from build123d import *

# Parameters (mm, degrees)
SKETCH_1_R          = 25
EXTRUDE_1_DEPTH     = 25
SKETCH_2_R          = 17.5
CUT_EXTRUDE_1_DEPTH = 10
SKETCH_3_R          = 2.5
CUT_EXTRUDE_2_DEPTH = 39.405728739


with BuildPart() as part:
    # 草图1 → 凸台-拉伸1 (new body)
    with BuildSketch(Plane(origin=(0, 0, 0), x_dir=(1, 0, 0), z_dir=(0, 1, 0))):
        with Locations(Location((0, 0, 0), (0, 0, 270))):
            Circle(SKETCH_1_R)
    extrude(amount=EXTRUDE_1_DEPTH)

    # 草图2 → 切除-拉伸1 (cut)
    with BuildSketch(Plane.XZ):
        with Locations(Location((0, 0, 0), (0, 0, 270))):
            Circle(SKETCH_2_R)
    cut_extrude_1 = extrude(amount=-CUT_EXTRUDE_1_DEPTH, mode=Mode.SUBTRACT)

    # 镜向1: 切除-拉伸1 across plane
    add(cut_extrude_1.mirror(Plane(origin=(0, 12.5, 0), x_dir=(0, 0, 1), z_dir=(0, -1, 0))), mode=Mode.SUBTRACT)

    # 草图3 → 切除-拉伸2 (cut, through all)
    with BuildSketch(Plane.XZ.offset(-10)):
        with Locations(Location((0, 0, 0), (0, 0, 270))):
            Circle(SKETCH_3_R)
    extrude(amount=-CUT_EXTRUDE_2_DEPTH, mode=Mode.SUBTRACT)


solid = part.part
Verification items for the finished model (mm, model axes). A direction names the side the tool comes from. Coordinates: 2 decimals unless noted, no trailing zeros. Write each loop counter-clockwise with the first axis right and the second up, starting at its lowest first coordinate (ties: lowest second). Pieces come first, ordered by that corner, then holes. Notation, with made-up numbers: (52.25, 54.25) - (98.25, 54.25) arc R26 cw to (98.25, 86.25) - close; hole circle Ø8 at (45.5, 48.25). An arc over 180 degrees is marked (long way). Answer as a JSON object with one key per item and string values.
(1) Cross-section at B-B on x = 0. Record the cut outline in (y, z).
Report:
{"outline": "(0, -25) - (25, -25) - (25, -17.5) - (15, -17.5) - (15, -2.5) - (10, -2.5) - (10, -17.5) - (0, -17.5) - close; (0, 17.5) - (10, 17.5) - (10, 2.5) - (15, 2.5) - (15, 17.5) - (25, 17.5) - (25, 25) - (0, 25) - close"}
(2) Cross-section at C-C on y = 12.5. Record the cut outline in (x, z).
Report:
{"outline": "circle Ø50 at (0, 0); hole circle Ø5 at (0, 0)"}
(3) Cross-section at A-A on z = 0. Record the cut outline in (x, y), plus the area to 3 significant figures.
Report:
{"outline": "(-25, 0) - (-17.5, 0) - (-17.5, 10) - (-2.5, 10) - (-2.5, 15) - (-17.5, 15) - (-17.5, 25) - (-25, 25) - close; (2.5, 10) - (17.5, 10) - (17.5, 0) - (25, 0) - (25, 25) - (17.5, 25) - (17.5, 15) - (2.5, 15) - close", "area": "525 mm^2"}
(4) Tool access check on faces 4 (the flat face through (-5, 25, -17)), 5 (the cylindrical face through (-10.648, 4.93, 13.887)), 6 (the cylindrical face through (-10.648, 20.07, 13.887)). Record the directions out of +Z, -Z, +X, -X, +Y, -Y that give a thin tool (end or side, any length) a straight path to the whole face; none if there is none.
Report:
{"face 4": "+Z, -Z, +X, -X, +Y", "face 5": "-Y", "face 6": "+Y"}
(5) Cross-section at D-D on x = -12. Record the cut outline in (y, z).
Report:
{"outline": "(0, -21.93) - (25, -21.93) - (25, -12.74) - (15, -12.74) - (15, 12.74) - (25, 12.74) - (25, 21.93) - (0, 21.93) - (0, 12.74) - (10, 12.74) - (10, -12.74) - (0, -12.74) - close"}
(6) Gauge pin test, flat ends, axial feed: pin 1 Ø6 at (x, y) = (-11, 8.5) entering from -Z; pin 2 Ø21 at (x, z) = (0, 0) entering from -Y; pin 3 Ø8 at (y, z) = (13, 19) entering from -X. Record the tip position at first contact, or that the pin passes through.
Report:
{"pin 1": "z = -23.69", "pin 2": "y = 10", "pin 3": "x = -20"}
(7) Thickness scan on line 1 along X through (y, z) = (3.5, 0); line 2 along Y through (x, z) = (13.5, -8); line 3 along X through (y, z) = (6, -12). Record the ranges inside material, lowest first.
Report:
{"line 1": "-25 to -17.5, 17.5 to 25", "line 2": "10 to 15", "line 3": "-21.93 to -12.74, 12.74 to 21.93"}
(8) Mould release check, pull along Z, two halves, no side actions. Record for faces 1 (the flat face through (-4, 10, 0)), 2 (the flat face through (-5, 0, -17)), 3 (the cylindrical face through (7.509, 12.325, 23.846)): pulls with the +Z half, pulls with the -Z half, needs draft (parallel to the pull), parting line crosses it, or undercut.
Report:
{"face 1": "undercut", "face 2": "needs draft", "face 3": "parting line crosses it"}
